Verification items for the finished model (mm, model axes). Face numbers are marked on the shaded views. A direction names the side the tool comes from. Coordinates: 2 decimals unless noted, no trailing zeros. Loops run counter-clockwise (first coordinate to the right, second up) from the corner with the lowest first, then second, coordinate; pieces in that order, holes last. Notation, with made-up numbers: (0, 42.5) -> (32, 42.5) arc R6 ccw to (32, 46.5) -> close; hole circle Ø1 at (-7, 31). An arc over 180 degrees is marked (long way). Answer as a JSON object with one key per item and string values. Group by question number.
Q1. Scan lines: L1, parallel to X at y = -150.5, z = 2.75; L2, parallel to Z at x = 42, y = -93; L3, parallel to Y at x = 54.5, z = 3.5. Record each from-to range of solid material in increasing order.
Q2. Gauge pin test, flat ends, axial feed: pin 1 Ø11.5 at (x, z) = (43.5, 7.5) entering from -Y; pin 2 Ø6 at (x, y) = (74, -40) entering from +Z; pin 3 Ø10 at (y, z) = (-173, 9.5) entering from +X. Record the tip position at first contact, or that the pin passes through.
Q3. Cross-section at D-D on x = 91.5. Record the boundary of the cut face in (y, z).
Q4. Cross-section at B-B on x = 59. Record the boundary of the cut face in (y, z).
Q5. Cross-section at A-A on z = 16.75. Record the boundary of the cut face in (x, y).
Q6. Cross-section at C-C on y = -27.5. Record the boundary of the cut face in (x, z).
Q7. Set-up check for the marked faces 1, 2 and 3: record each of +Z, -Z, +X, -X, +Y, -Y from which the full face is reachable in a straight line by a thin tool's end or side.
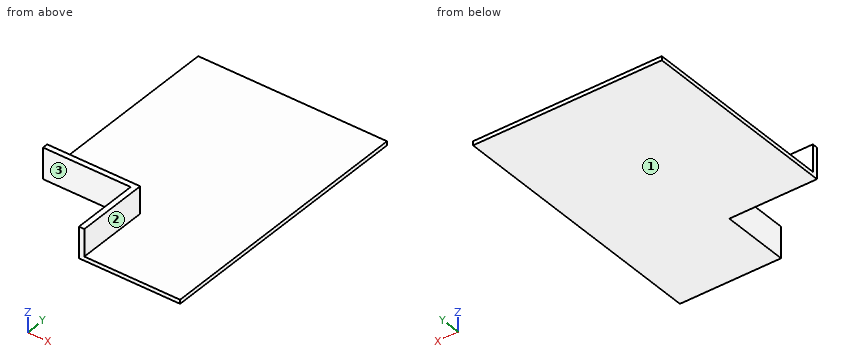
```python
from build123d import *

# Parameters (mm, degrees)
SKETCH_1_W          = 140
SKETCH_1_H          = 200
EXTRUDE_1_DEPTH     = 3
SKETCH_2_W          = 65
SKETCH_2_H          = 50
CUT_EXTRUDE_1_DEPTH = 10
SKETCH_3_W          = 4
SKETCH_3_H          = 50
EXTRUDE_2_DEPTH     = 23


with BuildPart() as part:
    # 草图1 → 凸台-拉伸1 (new body)
    with BuildSketch(Plane.XY):
        with Locations((70, -100)):
            Rectangle(SKETCH_1_W, SKETCH_1_H)
    extrude(amount=EXTRUDE_1_DEPTH)

    # 草图2 → 切除-拉伸1 (cut)
    with BuildSketch(Plane(origin=(0, 0, 0), x_dir=(-1, 0, 0), z_dir=(0, 0, -1))):
        with Locations((-32.5, -175)):
            Rectangle(SKETCH_2_W, SKETCH_2_H)
    extrude(amount=-CUT_EXTRUDE_1_DEPTH, mode=Mode.SUBTRACT)

    # 草图3 → 凸台-拉伸2 (add)
    with BuildSketch(Plane(origin=(0, 0, 0), x_dir=(-1, 0, 0), z_dir=(0, 0, -1))):
        with Locations((-67, -175)):
            Rectangle(SKETCH_3_W, SKETCH_3_H)
        Polygon((-65, -150), (0, -150), (0, -146), (-69, -146), (-69, -150), align=None)
    extrude(amount=-EXTRUDE_2_DEPTH)


solid = part.part
```
Computed values:
{
 "1": {"L1": "x = 65 to 140", "L2": "z = 0 to 3", "L3": "y = -150 to -146"},
 "2": {"pin 1": "stops at y = -150", "pin 2": "stops at z = 3", "pin 3": "stops at x = 69"},
 "3": {"outline": "(-200, 0) -> (0, 0) -> (0, 3) -> (-200, 3) -> close"},
 "4": {"outline": "(-150, 0) -> (0, 0) -> (0, 3) -> (-146, 3) -> (-146, 23) -> (-150, 23) -> close"},
 "5": {"outline": "(0, -150) -> (65, -150) -> (65, -200) -> (69, -200) -> (69, -146) -> (0, -146) -> close"},
 "6": {"outline": "(0, 0) -> (140, 0) -> (140, 3) -> (0, 3) -> close"},
 "7": {"face 1": "-Z, +X, -X, +Y, -Y", "face 2": "+Z, +X, +Y, -Y", "face 3": "+Z, -Z, -X, -Y"}
}
